from build123d import *

# Parameters (mm, degrees)
F1_DEPTH = 38.1
F3_DEPTH = 38.1


with BuildPart() as f1:
    # F0 (on Top) → F1 (new body)
    with BuildSketch(Plane.XY):
        with BuildLine():
            Line((609.6, 101.6), (609.6, 609.6))
            Line((609.6, 609.6), (-609.6, 609.6))
            Line((-609.6, 609.6), (-609.6, -609.6))
            Line((-609.6, -609.6), (-101.6, -609.6))
            Line((-101.6, -609.6), (-101.6, -245.284098))
            ThreePointArc((-101.6, -245.284098), (0, 0), (245.284098, 101.6))
            Line((245.284098, 101.6), (609.6, 101.6))
        make_face()
    extrude(amount=F1_DEPTH)

    # F2 (on face) → F3 (join)
    with BuildSketch(Plane(origin=(0, 0, 0), x_dir=(1, 0, 0), z_dir=(0, 0, -1))):
        Polygon((-197.565635, 125.723586), (-251.447171, 179.605122), (-538.815367, -107.763073), (-484.933831, -161.64461), align=None)
        Polygon((-161.64461, -484.933831), (-107.763073, -538.815367), (179.605122, -251.447171), (125.723586, -197.565635), align=None)
    extrude(amount=F3_DEPTH)


solid = f1.part
Can you work these out from the model? Positions are in its coordinate system, mm. A direction names the side the tool comes from. Coordinates: 2 decimals unless noted, no trailing zeros. Write each loop counter-clockwise with the first axis right and the second up, starting at its lowest first coordinate (ties: lowest second). Pieces come first, ordered by that corner, then holes. Notation, with made-up numbers: M -6.75,-25 L -0.75,-25 A28 ccw -0.75,-5 Z; hole C 85,16.5 d9. An arc over 180 degrees is marked long. Use one line per item in the form item = value.
Q1. I need wall thicknesses on line 1 along X through (y, z) = (-532, 19); line 2 along Z through (x, y) = (-204.5, -557); line 3 along Y through (x, z) = (275, 33.5). Which ranges of each line are inside material? Lowest first, please. Write a range as from..to.
Model answer:
line_1 = -609.6..-101.6
line_2 = 0..38.1
line_3 = 101.6..609.6
Q2. If we section it at C-C (y = -291): Write out the boundary of the cut face in (x, z), then the cut area to 3 significant figures.
Model answer:
outline = M -609.6,0 L -101.6,0 L -101.6,38.1 L -609.6,38.1 Z
area = 19,400 mm^2
Q3. If we section it at B-B (x = 29): Write out the boundary of the cut face in (y, z).
Model answer:
outline = M 25.92,0 L 294.29,0 L 294.29,-38.1 L 402.05,-38.1 L 402.05,0 L 609.6,0 L 609.6,38.1 L 25.92,38.1 Z
Q4. If we section it at D-D (y = 421): Write out the boundary of the cut face in (x, z), then the cut area to 3 significant figures.
Model answer:
outline = M -609.6,0 L -97.71,0 L -97.71,-38.1 L 10.05,-38.1 L 10.05,0 L 609.6,0 L 609.6,38.1 L -609.6,38.1 Z
area = 50,600 mm^2
Q5. If we section it at A-A (z = -19): Write out the boundary of the cut face in (x, y), then the cut area to 3 significant figures.
Model answer:
outline = M -538.82,107.76 L -251.45,-179.61 L -197.57,-125.72 L -484.93,161.64 Z; M -161.64,484.93 L 125.72,197.57 L 179.61,251.45 L -107.76,538.82 Z
area = 61,900 mm^2
Q6. For faces 1 (the flat face through (-101.6, -430, 19)), 2 (the flat face through (-224.13, -152.29, -18.78)), 3 (the flat face through (-144, 144, 0)), 4 (the flat face through (33.91, 397.14, -18.78)), 5 (the flat face through (-393.12, -37.93, -18.78)), which set-ups out of +Z, -Z, +X, -X, +Y, -Y let a thin tool reach every point of the face, with its end or its side?
Model answer:
face_1 = +Z, -Z, +X, -Y
face_2 = -Z, +X, -Y
face_3 = -Z
face_4 = -Z, +X, +Y
face_5 = -Z, -X, -Y
Q7. For P1, Ø5, axis at x = 278, z = 10, coming from the -Y side; P2, Ø1, axis at x = -350, z = -9, coming from the -Y side; P3, Ø4, axis at y = 131.5, z = -26, coming from the -X side, each with a flat end and sliding along its axis, tell me the tip position at first contact or that it passes through.
Model answer:
P1 = 101.6
P2 = -81.55
P3 = -517.08
